Source: CAD feature listing. Evaluate the final solid. Frame: model axes, mm. Face numbers are marked on the shaded views. Give positions to 0.01 mm unless a question says otherwise; leave off trailing zeros. Order: outer loops, then holes, each group sorted by start corner. A loop starts at its lowest first (then second) coordinate and runs counter-clockwise, first axis right, second up. Notation, with made-up numbers: (-36.5, 18) -> (-27.5, 18) arc R9 cw to (-27.5, 23) -> close; hole circle Ø6 at (-7, -18.5). An arc over 180 degrees is marked (long way). Use CSV: the item, a comma, the result in double quotes.
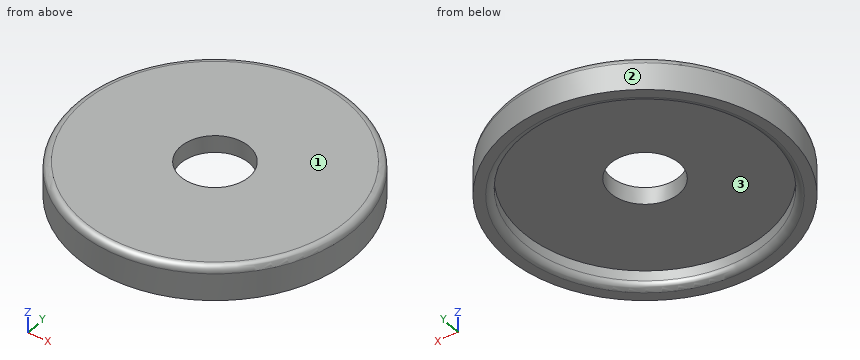
```python
from build123d import *

# Parameters (mm, degrees)
F0_R     = 45.24375
F0_R_2   = 12.7
F1_DEPTH = 6.35
F0_R_3   = 51.59375
F2_DEPTH = 12.7
F3_R     = 2.54
F4_R     = 2.54


with BuildPart() as f1:
    # F0 (on Top) → F1 (new body)
    with BuildSketch(Plane.XY):
        Circle(F0_R)
        Circle(F0_R_2, mode=Mode.SUBTRACT)
    extrude(amount=-F1_DEPTH)

    # F0 (on Top) → F2 (join)
    with BuildSketch(Plane.XY):
        Circle(F0_R_3)
        Circle(F0_R, mode=Mode.SUBTRACT)
    extrude(amount=-F2_DEPTH)

    # F3
    f3_edges = [f1.edges().sort_by_distance(p)[0] for p in [
        (-51.59375, 0, 0),
    ]]
    fillet(f3_edges, radius=F3_R)

    # F4
    f4_edges = [f1.edges().sort_by_distance(p)[0] for p in [
        (-45.24375, 0, -12.7),
    ]]
    fillet(f4_edges, radius=F4_R)


solid = f1.part
```
1. Section query D-D on z = -1.25. Return loops of the section in (x, y).
Answer below:
outline,"circle Ø102.48 at (0, 0); hole circle Ø25.4 at (0, 0)"
2. Section query A-A on y = 0. Return loops of the section in (x, z).
Answer below:
outline,"(-51.59, -12.7) -> (-47.78, -12.7) arc R2.54 ccw to (-45.24, -10.16) -> (-45.24, -6.35) -> (-12.7, -6.35) -> (-12.7, 0) -> (-49.05, 0) arc R2.54 ccw to (-51.59, -2.54) -> close; (12.7, -6.35) -> (45.24, -6.35) -> (45.24, -10.16) arc R2.54 ccw to (47.78, -12.7) -> (51.59, -12.7) -> (51.59, -2.54) arc R2.54 ccw to (49.05, 0) -> (12.7, 0) -> close"
3. Mould query, pull axis X, two halves, no side actions, for the marked faces 1, 2 and 3. Classes: released by +X, released by -X, zero draft, split by the parting line, or undercut.
Answer below:
face 1,"zero draft"
face 2,"split by the parting line"
face 3,"undercut"
4. Ray query, line 1 along Y through (x, z) = (0, -7.35); line 2 along Y through (x, z) = (0, -4.25); line 3 along Z through (x, y) = (-20, -32.5). Return the intervals inside material, ascending.
Answer below:
line 1,"y = -51.59 to -45.24, 45.24 to 51.59"
line 2,"y = -51.59 to -12.7, 12.7 to 51.59"
line 3,"z = -6.35 to 0"
5. Pin query (flat end, axial travel): P1, Ø5, axis at x = -38.5, z = -10, coming from the -Y side; P2, Ø1, axis at x = -35.5, y = -8, coming from the -Z side; P3, Ø2, axis at x = -27.5, z = -10.5, coming from the -Y side; P4, Ø6, axis at x = 27.5, y = -7.5, coming from the +Z side. Return the tip coordinate at first contact, or that it passes through.
Answer below:
P1,"stops at y = -36.96"
P2,"stops at z = -6.35"
P3,"stops at y = -44.27"
P4,"stops at z = 0"
6. Section query C-C on z = -8.5. Return loops of the section in (x, y), plus the area to 3 significant figures.
Answer below:
outline,"circle Ø103.19 at (0, 0); hole circle Ø90.49 at (0, 0)"
area,"1,930 mm²"
